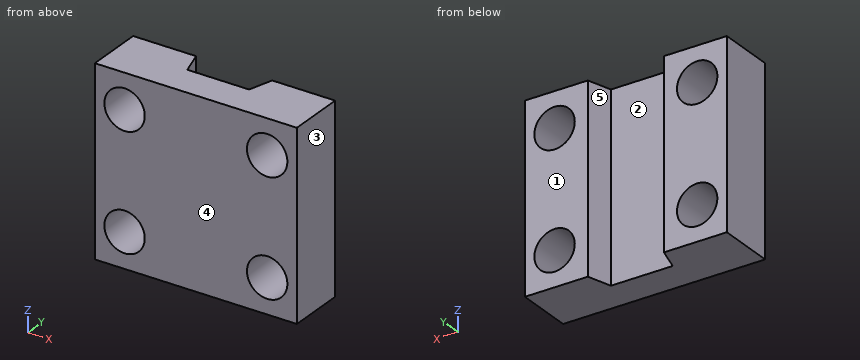
Autodesk Inventor part; units mm, degrees
sketch "Эскиз1" plane through (0, 0, 0) normal (0, 1, 0) x (-1, 0, 0)
  line L0 (21.25, 19.5) -> (-21.25, 19.5)
  line L1 (-21.25, 19.5) -> (-21.25, -19.5)
  line L2 (-21.25, -19.5) -> (21.25, -19.5)
  line L3 (21.25, -19.5) -> (21.25, 19.5)
  line L4 (21.25, 19.5) -> (-21.25, -19.5) construction
  line L5 (-21.25, 19.5) -> (21.25, -19.5) construction
  circle A0 centre (-15, -12.15) radius 4.25
  line L6 (0, -19.5) -> (0, 19.5) construction
  line L7 (-21.25, 0) -> (21.25, 0) construction
  circle A1 centre (15, -12.15) radius 4.25
  circle A2 centre (-15, 12.15) radius 4.25
  circle A3 centre (15, 12.15) radius 4.25
  point P0 (0, 0)
  dimension "d0" = 39
  dimension "d1" = 42.5
  dimension "d2" = 8.5
  dimension "d3" = 6.25
  dimension "d4" = 7.35
extrude "Выдавливание1" add sketch "Эскиз1" along normal blind 12
sketch "Эскиз2" plane through (-21.25, 0, 19.5) normal (0, 0, 1) x (1, 0, 0)
  line L0 (14.75, 7) -> (27.75, 7)
  line L1 (0, 12) -> (42.5, 12)
  line L2 (13.25, 12) -> (29.25, 12)
  line L3 (21.25, 14.4) -> (21.25, -2.4) construction
  line L4 (13.25, 12) -> (14.75, 7)
  line L5 (29.25, 12) -> (27.75, 7)
  point P0 (21.25, 0)
  point P1 (21.25, 12)
  point P2 (21.25, 7)
  point P3 (13.25, 12)
  dimension "d7" = 13
  dimension "d8" = 5
  dimension "d9" = 16
extrude "Выдавливание2" cut sketch "Эскиз2" against normal up to surface (39 mm away)
properties part number "Крепление мотора2"
Model file for the job. Use its own axes, mm. Face numbers are marked on the shaded views. A direction names the side the tool comes from. Round coordinates to 2 decimals unless told otherwise and drop trailing zeros. Write each loop counter-clockwise with the first axis right and the second up, starting at its lowest first coordinate (ties: lowest second). Pieces come first, ordered by that corner, then holes. Notation, with made-up numbers: (-33.75, 63.5) -> (-6.75, 63.5) arc R29 cw to (-6.75, 92.5) -> close; hole circle Ø11 at (47.5, -33). An arc over 180 degrees is marked (long way). Answer as CSV lines item,"result".
1. Tool access for the marked faces 1 and 2: list every direction of +Z, -Z, +X, -X, +Y, -Y with a clear straight run to the whole face (end or side of a thin tool).
Resolved:
face 1,"+Z, -Z, +X, -X, +Y"
face 2,"+Z, -Z, +Y"
2. Slice it at C-C, the plane y = 2.5. List the corners of the cut face in (x, z).
Resolved:
outline,"(-21.25, -19.5) -> (21.25, -19.5) -> (21.25, 19.5) -> (-21.25, 19.5) -> close; hole circle Ø8.5 at (-15, -12.15); hole circle Ø8.5 at (-15, 12.15); hole circle Ø8.5 at (15, -12.15); hole circle Ø8.5 at (15, 12.15)"
3. Drill centre lines: line 1 (X direction, y = 4.5, z = -12); line 2 (Z direction, x = -15, y = 7); line 3 (Z direction, x = -17.5, y = 7.25). Where is each one in solid material? Low to high.
Resolved:
line 1,"-21.25 to -19.25, -10.75 to 10.75, 19.25 to 21.25"
line 2,"-19.5 to -16.4, -7.9 to 7.9, 16.4 to 19.5"
line 3,"-19.5 to -15.59, -8.71 to 8.71, 15.59 to 19.5"
4. Slice it at B-B, the plane x = -13. List the corners of the cut face in (y, z).
Resolved:
outline,"(0, -19.5) -> (12, -19.5) -> (12, -15.9) -> (0, -15.9) -> close; (0, -8.4) -> (12, -8.4) -> (12, 8.4) -> (0, 8.4) -> close; (0, 15.9) -> (12, 15.9) -> (12, 19.5) -> (0, 19.5) -> close"
5. Slice it at A-A, the plane z = -12.15. List the corners of the cut face in (x, y), plus the area to 4 significant figures.
Resolved:
outline,"(-21.25, 0) -> (-19.25, 0) -> (-19.25, 12) -> (-21.25, 12) -> close; (-10.75, 0) -> (10.75, 0) -> (10.75, 12) -> (8, 12) -> (6.5, 7) -> (-6.5, 7) -> (-8, 12) -> (-10.75, 12) -> close; (19.25, 0) -> (21.25, 0) -> (21.25, 12) -> (19.25, 12) -> close"
area,"233.5 mm²"
6. Slice it at D-D, the plane y = 9.25. List the corners of the cut face in (x, z) (3 decimals), plus the area to 3 significant figures.
Resolved:
outline,"(-21.25, -19.5) -> (-7.175, -19.5) -> (-7.175, 19.5) -> (-21.25, 19.5) -> close; (7.175, -19.5) -> (21.25, -19.5) -> (21.25, 19.5) -> (7.175, 19.5) -> close; hole circle Ø8.5 at (-15, -12.15); hole circle Ø8.5 at (-15, 12.15); hole circle Ø8.5 at (15, -12.15); hole circle Ø8.5 at (15, 12.15)"
area,"871 mm²"
7. Mould opens along X. For the marked faces 3, 4 and 5 say: +X half, -X half, draft (parallel to the pull), parting line (faces both ways), or undercut.
Resolved:
face 3,"+X half"
face 4,"draft"
face 5,"undercut"
